Job drawing, mm, ordinate dimensions from the low corner. One solid piece. A direction names the side the tool comes from. Round coordinates to 2 decimals unless told otherwise and drop trailing zeros. Write each loop counter-clockwise with the first axis right and the second up, starting at its lowest first coordinate (ties: lowest second). Pieces come first, ordered by that corner, then holes. Notation, with made-up numbers: (86, 6.5) - (120, 6.5) arc R13 ccw to (120, 20.5) - close; hole circle Ø6 at (82.5, -2.75). An arc over 180 degrees is marked (long way). Write each question's results on one line, items separated by ' | '.
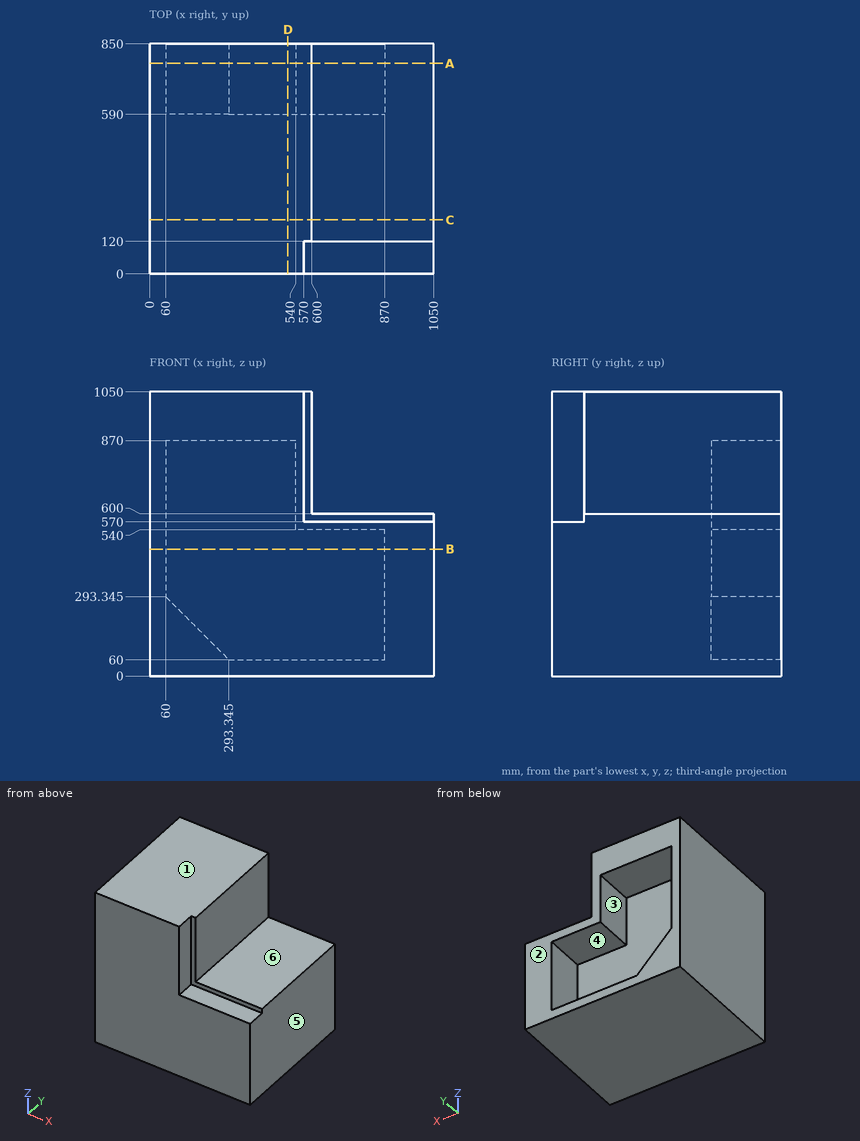
(1) Slice it at B-B, the plane z = 469. Write the cut outline in (x, y).
Worked answers:
outline: (0, 0) - (1050, 0) - (1050, 850) - (870, 850) - (870, 590) - (60, 590) - (60, 850) - (0, 850) - close
(2) Slice it at D-D, the plane x = 511.5. Write the cut outline in (y, z).
Worked answers:
outline: (0, 0) - (850, 0) - (850, 60) - (590, 60) - (590, 870) - (850, 870) - (850, 1050) - (0, 1050) - close
(3) Slice it at C-C, the plane y = 200. Write the cut outline in (x, z), and give its area (3 significant figures).
Worked answers:
outline: (0, 0) - (1050, 0) - (1050, 600) - (600, 600) - (600, 1050) - (0, 1050) - close | area: 900,000 mm2
(4) Drill centre lines: probe 1 along X at (y, z) = (608.5, 393); probe 2 along X at (y, z) = (803.5, 602.5); probe 3 along Z at (x, y) = (604, 262.5). Where is each one in solid material? Low to high. Write a range as [from, to].
Worked answers:
probe 1: x = [0, 60], [870, 1050] | probe 2: x = [0, 60], [540, 600] | probe 3: z = [0, 600]
(5) Flat gauge pin, fed straight in: pin 1 Ø6 at (x, y) = (682, 175) entering from +Z. Where does the tip first touch, or does it go through?
Worked answers:
pin 1: stops at z = 600
(6) Tool access for the marked faces 4, 5 and 6: list every direction of +Z, -Z, +X, -X, +Y, -Y with a clear straight run to the whole face (end or side of a thin tool).
Worked answers:
face 4: +Y | face 5: +Z, -Z, +X, +Y, -Y | face 6: +Z, +X, +Y, -Y
(7) Slice it at A-A, the plane y = 778.5. Write the cut outline in (x, z) (1 decimal), and give its area (3 significant figures).
Worked answers:
outline: (0, 0) - (1050, 0) - (1050, 600) - (600, 600) - (600, 1050) - (0, 1050) - close; hole (60, 293.3) - (293.3, 60) - (870, 60) - (870, 540) - (540, 540) - (540, 870) - (60, 870) - close | area: 380,000 mm2
(8) Two-plate mould, pull along Z, no slides. Class the marked faces 1, 2 and 3: released by +Z, released by -Z, zero draft, split by the parting line, or undercut.
Worked answers:
face 1: released by +Z | face 2: zero draft | face 3: undercut
